```python
from build123d import *

# Parameters (mm, degrees)
SKETCH2_R           = 1.35
BOSS_EXTRUDE1_DEPTH = 3
CIRPATTERN1_COUNT   = 6
CUT_EXTRUDE3_DEPTH  = 5
CUT_EXTRUDE9_DEPTH  = 10


with BuildPart() as part:
    # Sketch2 → Boss-Extrude1 (new body)
    with BuildSketch(Plane(origin=(0, 0, 0), x_dir=(1, 0, 0), z_dir=(0, 1, 0))):
        Polygon((0, 125), (-58.08143708, 125), (-35.58143708, 86.02885683), (-56.712456933, 73.82885683), (-79.212456933, 112.8), (-108.253175473, 62.5), (0, 0), align=None)
        with Locations(Location((-37.385731074, 81.753985699, 0), (0, 0, 270))):
            Circle(SKETCH2_R, mode=Mode.SUBTRACT)
        with Locations(Location((-52.108162939, 73.253985699, 0), (0, 0, 270))):
            Circle(SKETCH2_R, mode=Mode.SUBTRACT)
        with Locations(Location((-60.887328063, 75.459945743, 0), (0, 0, 270))):
            Circle(SKETCH2_R, mode=Mode.SUBTRACT)
        with Locations(Location((-34.90656595, 90.459945743, 0), (0, 0, 270))):
            Circle(SKETCH2_R, mode=Mode.SUBTRACT)
        with Locations(Location((-51.90656595, 119.904809472, 0), (0, 0, 270))):
            Circle(SKETCH2_R, mode=Mode.SUBTRACT)
        with Locations(Location((-43.40656595, 105.182377607, 0), (0, 0, 270))):
            Circle(SKETCH2_R, mode=Mode.SUBTRACT)
        with Locations(Location((-69.387328063, 90.182377607, 0), (0, 0, 270))):
            Circle(SKETCH2_R, mode=Mode.SUBTRACT)
        with Locations(Location((-77.887328063, 104.904809472, 0), (0, 0, 270))):
            Circle(SKETCH2_R, mode=Mode.SUBTRACT)
    boss_extrude1 = extrude(amount=BOSS_EXTRUDE1_DEPTH)

    # CirPattern1: Boss-Extrude1 ×6 about axis
    cirpattern1_axis = Axis((0, 0, 0), (0, 1, 0))
    for i in range(1, CIRPATTERN1_COUNT):
        add(boss_extrude1.rotate(cirpattern1_axis, i * 360 / CIRPATTERN1_COUNT))

    # Sketch4 → Cut-Extrude3 (cut)
    with BuildSketch(Plane(origin=(0, 3, 0), x_dir=(1, 0, 0), z_dir=(0, 1, 0))):
        with BuildLine():
            Line((79.212456933, -112.8), (137.293894013, -12.2))
            ThreePointArc((137.293894013, -12.2), (125.5592118, -23.716902798), (109.56410095, -27.524558982))
            ThreePointArc((109.56410095, -27.524558982), (77.942286341, -45), (78.619017782, -81.123015275))
            ThreePointArc((78.619017782, -81.123015275), (83.319046223, -96.879015699), (79.212456933, -112.8))
        make_face()
        with BuildLine():
            Line((137.293894013, 12.2), (79.212456933, 112.8))
            ThreePointArc((79.212456933, 112.8), (83.319046223, 96.879015699), (78.619017782, 81.123015275))
            ThreePointArc((78.619017782, 81.123015275), (77.942286341, 45), (109.56410095, 27.524558982))
            ThreePointArc((109.56410095, 27.524558982), (125.5592118, 23.716902798), (137.293894013, 12.2))
        make_face()
        with BuildLine():
            Line((58.08143708, 125), (-58.08143708, 125))
            ThreePointArc((-58.08143708, 125), (-42.240165578, 120.595918497), (-30.945083169, 108.647574257))
            ThreePointArc((-30.945083169, 108.647574257), (0, 90), (30.945083169, 108.647574257))
            ThreePointArc((30.945083169, 108.647574257), (42.240165578, 120.595918497), (58.08143708, 125))
        make_face()
        with BuildLine():
            Line((-79.212456933, 112.8), (-137.293894013, 12.2))
            ThreePointArc((-137.293894013, 12.2), (-125.5592118, 23.716902798), (-109.56410095, 27.524558982))
            ThreePointArc((-109.56410095, 27.524558982), (-77.942286341, 45), (-78.619017782, 81.123015275))
            ThreePointArc((-78.619017782, 81.123015275), (-83.319046223, 96.879015699), (-79.212456933, 112.8))
        make_face()
        with BuildLine():
            Line((-137.293894013, -12.2), (-79.212456933, -112.8))
            ThreePointArc((-79.212456933, -112.8), (-83.319046223, -96.879015699), (-78.619017782, -81.123015275))
            ThreePointArc((-78.619017782, -81.123015275), (-77.942286341, -45), (-109.56410095, -27.524558982))
            ThreePointArc((-109.56410095, -27.524558982), (-125.5592118, -23.716902798), (-137.293894013, -12.2))
        make_face()
        with BuildLine():
            Line((-58.08143708, -125), (58.08143708, -125))
            ThreePointArc((58.08143708, -125), (42.240165578, -120.595918497), (30.945083169, -108.647574257))
            ThreePointArc((30.945083169, -108.647574257), (0, -90), (-30.945083169, -108.647574257))
            ThreePointArc((-30.945083169, -108.647574257), (-42.240165578, -120.595918497), (-58.08143708, -125))
        make_face()
    extrude(amount=-CUT_EXTRUDE3_DEPTH, mode=Mode.SUBTRACT)

    # Sketch8 → Cut-Extrude9 (cut)
    with BuildSketch(Plane(origin=(0, 3, 0), x_dir=(1, 0, 0), z_dir=(0, 1, 0))):
        with BuildLine():
            Line((-79.627397697, 112.081427342), (-137.090413308, 12.563994028))
            ThreePointArc((-137.090413308, 12.563994028), (-131.312677504, 18.215244412), (-123.44128918, 20.048304088))
            ThreePointArc((-123.44128918, 20.048304088), (-77.942300503, 45.000018775), (-79.083064161, 96.879154221))
            ThreePointArc((-79.083064161, 96.879154221), (-81.425302856, 104.406169658), (-79.627397697, 112.081427342))
        make_face()
        with BuildLine():
            Line((-136.879097611, -12.918653567), (-79.425980046, -112.441801521))
            ThreePointArc((-79.425980046, -112.441801521), (-81.43123854, -104.612510346), (-79.083020624, -96.879158257))
            ThreePointArc((-79.083020624, -96.879158257), (-77.942345072, -45.000020873), (-123.441376125, -20.048383457))
            ThreePointArc((-123.441376125, -20.048383457), (-131.131082054, -18.31331395), (-136.879097611, -12.918653567))
        make_face()
        with BuildLine():
            Line((-57.251702025, -125.000120556), (57.66443115, -125.005835196))
            ThreePointArc((57.66443115, -125.005835196), (49.881436852, -122.827794405), (44.358266444, -116.927501992))
            ThreePointArc((44.358266444, -116.927501992), (-4.6681e-05, -90.000079294), (-44.358314075, -116.927577326))
            ThreePointArc((-44.358314075, -116.927577326), (-49.70578131, -122.719523255), (-57.251702025, -125.000120556))
        make_face()
        with BuildLine():
            Line((79.627393474, -112.081506636), (137.090409084, -12.564073322))
            ThreePointArc((137.090409084, -12.564073322), (131.312673281, -18.215323706), (123.441284957, -20.048383382))
            ThreePointArc((123.441284957, -20.048383382), (77.94229628, -45.000098069), (79.083059938, -96.879233516))
            ThreePointArc((79.083059938, -96.879233516), (81.425298632, -104.406248952), (79.627393474, -112.081506636))
        make_face()
        with BuildLine():
            Line((136.879093387, 12.918574273), (79.425975823, 112.441722226))
            ThreePointArc((79.425975823, 112.441722226), (81.431234317, 104.612431052), (79.083016401, 96.879078963))
            ThreePointArc((79.083016401, 96.879078963), (77.942340849, 44.999941578), (123.441371902, 20.048304163))
            ThreePointArc((123.441371902, 20.048304163), (131.131077831, 18.313234656), (136.879093387, 12.918574273))
        make_face()
        with BuildLine():
            Line((57.251697801, 125.000041262), (-57.664435373, 125.005755901))
            ThreePointArc((-57.664435373, 125.005755901), (-49.881441076, 122.827715111), (-44.358270668, 116.927422698))
            ThreePointArc((-44.358270668, 116.927422698), (4.2458e-05, 90), (44.358309852, 116.927498031))
            ThreePointArc((44.358309852, 116.927498031), (49.705777087, 122.71944396), (57.251697801, 125.000041262))
        make_face()
    extrude(amount=-CUT_EXTRUDE9_DEPTH, mode=Mode.SUBTRACT)


solid = part.part
```
Work out the finished part from the listing and answer in its coordinate system (mm). A direction names the side the tool comes from. Give positions to 0.01 mm unless a question says otherwise; leave off trailing zeros. Write each loop counter-clockwise with the first axis right and the second up, starting at its lowest first coordinate (ties: lowest second). Pieces come first, ordered by that corner, then holes. Notation, with made-up numbers: (-36, -35.75) - (-30, -35.75) arc R29 ccw to (-30, 3.25) - close; hole circle Ø9 at (-39.75, 2). An arc over 180 degrees is marked (long way). Use one line per item in the form item = value.
1. A cutting plane is placed at C-C (y = 1.35). State how many separate pieces and enclosed holes the cut face has, and give its area (3 significant figures).
Filled in:
separate_pieces = 1
enclosed_holes = 48
area = 31,900 mm^2
2. For faces 4 (the face through (-25.68, 1.52, 97.1)), 5 (the face through (-49.46, 1.52, -122.56)), 6 (the face through (-46.295, 1.479, 79.843)), 7 (the face through (-71.25, 1.52, -70.75)), determine the directions among +Z, -Z, +X, -X, +Y, -Y from which every point of the face is accessible in a straight line to the end or side of a thin tool.
Filled in:
face_4 = +Z, +Y, -Y
face_5 = -Z, +Y, -Y
face_6 = +Y, -Y
face_7 = -X, +Y, -Y
3. Consider L1, parallel to Z at x = 120, y = 1.4; L2, parallel to X at y = 1.25, z = 81; L3, parallel to X at y = 2.55, z = -89. Determine where each line is inside the solid, lowest interval first.
Filled in:
L1 = -20.02 to -12.2, 12.2 to 20.02
L2 = -72.47 to -60.85, -44.29 to -38.51, -36.27 to 36.27, 38.51 to 44.29, 60.85 to 72.47
L3 = -74.99 to -70.04, -68.74 to -65.47, -37.3 to 37.3, 65.47 to 68.74, 70.04 to 74.99
4. A cutting plane is placed at B-B (x = -7.5). Write down the section's boundary in (y, z), and give its area (3 significant figures).
Filled in:
outline = (0, -90.57) - (3, -90.57) - (3, 90.57) - (0, 90.57) - close
area = 543 mm^2
5. This flat-tipped pin is pushed along its axis until it touches: pin 1 Ø1 at (y, z) = (1, -10) entering from +X. Where does it stop, or does it pass through?
Filled in:
pin_1 = 92.29
6. A cutting plane is placed at A-A (z = 2.5). Write down the section's boundary in (x, y), and give its area (3 significant figures).
Filled in:
outline = (-92.29, 0) - (92.29, 0) - (92.29, 3) - (-92.29, 3) - close
area = 554 mm^2
7. Determine the mould class of faces 1 (the face through (-68.12, 1.48, 93.59)), 2 (the face through (71.25, 1.52, 70.78)), 3 (the face through (1, 3, -3)) for opening direction X: released by +X, released by -X, zero draft, split by the parting line, or undercut.
Filled in:
face_1 = undercut
face_2 = released by +X
face_3 = zero draft
